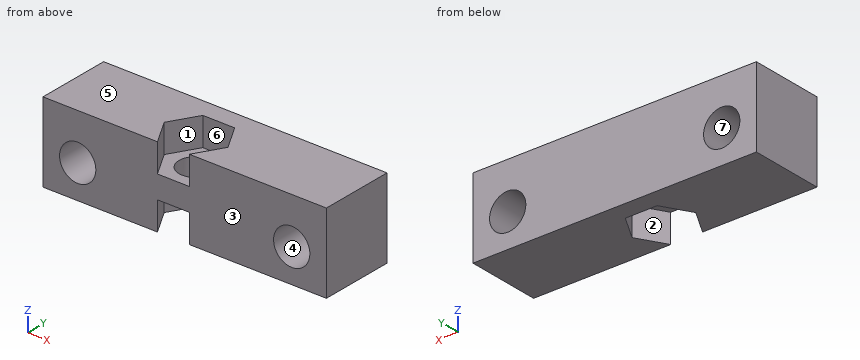
from build123d import *

# Parameters (mm, degrees)
SKETCH1_W               = 25
SKETCH1_H               = 7
SKETCH1_R               = 1.6
BOSS_EXTRUDE1_DEPTH     = 6.5
CUT_EXTRUDE1_START      = -1
SKETCH3_R               = 1.5
CUT_EXTRUDE1_DEPTH      = 15.386682553
CUT_EXTRUDE2_START      = 1
CUT_EXTRUDE2_OUTLINE_R  = 1.5
CUT_EXTRUDE2_DEPTH      = 2.5
CUT_EXTRUDE3_DEPTH      = 16.386682553
CUT_EXTRUDE3_DEPTH_BACK = 16.386682553
SKETCH3_3_R             = 1.5


# Read off the part's stored shape, not the designer's step: Cut-Extrude2
with BuildPart() as part:
    # Sketch1 → Boss-Extrude1 (new body)
    with BuildSketch(Plane(origin=(0, 0, 0), x_dir=(1, 0, 0), z_dir=(0, 1, 0))):
        with Locations((1, 0)):
            Rectangle(SKETCH1_W, SKETCH1_H)
        with Locations(Location((10.44, 0.56, 0), (0, 0, 90))):
            Circle(SKETCH1_R, mode=Mode.SUBTRACT)
        with Locations(Location((-8.44, 0.56, 0), (0, 0, 90))):
            Circle(SKETCH1_R, mode=Mode.SUBTRACT)
    extrude(amount=BOSS_EXTRUDE1_DEPTH)

    # Sketch3 → Cut-Extrude1 (cut, through all)
    with BuildSketch(Plane.XY.offset(CUT_EXTRUDE1_START)):
        Polygon((1.405847905, 0), (2.811695811, 2.435), (1.405847905, 4.87), (-1.405847905, 4.87), (-2.811695811, 2.435), (-1.405847905, 0), align=None)
        with Locations((0, 2.435)):
            Circle(SKETCH3_R, mode=Mode.SUBTRACT)
    extrude(amount=-CUT_EXTRUDE1_DEPTH, mode=Mode.SUBTRACT)

    # Cut-Extrude2 outline → Cut-Extrude2 (cut)
    with BuildSketch(Plane.XY.offset(CUT_EXTRUDE2_START)):
        Polygon((-2.811695811, 2.435), (-1.405847905, 0), (1.405847905, 0), (2.811695811, 2.435), (1.405847905, 4.87), (-1.405847905, 4.87), align=None)
        with Locations((0, 2.435)):
            Circle(CUT_EXTRUDE2_OUTLINE_R, mode=Mode.SUBTRACT)
    extrude(amount=CUT_EXTRUDE2_DEPTH, mode=Mode.SUBTRACT)

    # Sketch3<3> → Cut-Extrude3 (cut, two sides: drawn at the far end of the back side and taken through both)
    with BuildSketch(Plane.XY.offset(-CUT_EXTRUDE3_DEPTH_BACK)):
        with Locations((0, 2.435)):
            Circle(SKETCH3_3_R)
    extrude(amount=CUT_EXTRUDE3_DEPTH + CUT_EXTRUDE3_DEPTH_BACK, mode=Mode.SUBTRACT)


solid = part.part
The listing builds one solid part. Answer for the finished solid, in the listing's coordinates (mm). Face numbers are marked on the shaded views. A direction names the side the tool comes from. Round coordinates to 2 decimals unless told otherwise and drop trailing zeros. Write each loop counter-clockwise with the first axis right and the second up, starting at its lowest first coordinate (ties: lowest second). Pieces come first, ordered by that corner, then holes. Notation, with made-up numbers: M 60,47.5 L 86,47.5 A10 cw 86,58.5 Z; hole C 39.5,56.25 d3. An arc over 180 degrees is marked long. Write each question's results on one line, items separated by ' | '. Start each with the question number.
Item 1: Straight lines are drawn through the part: L1, parallel to X at y = 4.25, z = -0.75; L2, parallel to Z at x = -8.44, y = 4; L3, parallel to X at y = 0.75, z = -1.25. For each, find the intervals that lie inside material, in ascending order. Write a range as [from, to].
Item 2: For a pull along Z with two mould halves and no side action, classify the marked faces 4, 5, 6 and 7 as pulls with the +Z half, pulls with the -Z half, needs draft (parallel to the pull), parting line crosses it, or undercut.
Item 3: A cutting plane is placed at B-B on z = -1.5. Write down the section's boundary in (x, y) (3 decimals), and give its area (3 significant figures).
Item 4: A cutting plane is placed at A-A on x = 10.44. Write down the section's boundary in (y, z), and give its area (3 significant figures).
Item 5: For the marked faces 1, 2 and 3, determine the directions among +Z, -Z, +X, -X, +Y, -Y from which every point of the face is accessible in a straight line to the end or side of a thin tool.
Item 6: A cutting plane is placed at C-C on y = 5.5. Write down the section's boundary in (x, z), and give its area (3 significant figures).
Item 7: A flat-ended cylindrical pin translates along its axis: pin 1 Ø1.5 at (x, y) = (1, 2) entering from +Z. Find the tip coordinate at first contact, or state that the pin passes through.
Item 8: A cutting plane is placed at D-D on z = -0.25. Write down the section's boundary in (x, y) (3 decimals).
Check sheet entries:
1) L1: [-11.5, -10.03], [-6.85, 8.85], [12.03, 13.5] | L2: [-3.5, -2.16], [1.04, 3.5] | L3: [-11.5, -9.88], [-7, -1.84], [1.84, 9], [11.88, 13.5]
2) face 4: undercut | face 5: pulls with the +Z half | face 6: needs draft | face 7: undercut
3) outline: M -11.5,0 L -9.735,0 L -9.735,6.5 L -11.5,6.5 Z; M -7.145,0 L -1.406,0 L -2.812,2.435 L -1.406,4.87 L 1.406,4.87 L 2.812,2.435 L 1.406,0 L 9.145,0 L 9.145,6.5 L -7.145,6.5 Z; M 11.735,0 L 13.5,0 L 13.5,6.5 L 11.735,6.5 Z | area: 108 mm²
4) outline: M 0,-3.5 L 6.5,-3.5 L 6.5,-2.16 L 0,-2.16 Z; M 0,1.04 L 6.5,1.04 L 6.5,3.5 L 0,3.5 Z | area: 24.7 mm²
5) face 1: +Z | face 2: -Z | face 3: +Z, -Z, +X, -X, -Y
6) outline: M -11.5,-3.5 L 13.5,-3.5 L 13.5,3.5 L -11.5,3.5 Z; hole C -8.44,-0.56 d3.2; hole C 10.44,-0.56 d3.2 | area: 159 mm²
7) pin 1: z = 1
8) outline: M -11.5,0 L -10.01,0 L -10.01,6.5 L -11.5,6.5 Z; M -6.87,0 L 8.87,0 L 8.87,6.5 L -6.87,6.5 Z; M 12.01,0 L 13.5,0 L 13.5,6.5 L 12.01,6.5 Z; hole C 0,2.435 d3
